Design review of the part built by this model. Coordinates are the model's own, in mm. A direction names the side the tool comes from. Coordinates: 2 decimals unless noted, no trailing zeros. Write each loop counter-clockwise with the first axis right and the second up, starting at its lowest first coordinate (ties: lowest second). Pieces come first, ordered by that corner, then holes.
```python
from build123d import *

# Parameters (mm, degrees)
SZKIC3_W                    = 1
SZKIC3_H                    = 17.528511895
WYTNIJ_WYCI_GNI_CIE1_DEPTH  = 35
WYTNIJ_WYCI_GNI_CIE4_DEPTH  = 12
SZKIC10_R                   = 6.25
DODANIE_WYCI_GNI_CIE5_DEPTH = 8
WYTNIJ_WYCI_GNI_CIE5_DEPTH  = 5
SZKIC12_R                   = 4
DODANIE_WYCI_GNI_CIE6_DEPTH = 23


with BuildPart() as part:
    # Szkic2 → Obrót1 (revolve)
    with BuildSketch(Plane(origin=(0, 0, 0), x_dir=(1, 0, 0), z_dir=(0, 1, 0))):
        Polygon((0, 0), (0, -40), (7, -53), (7, -63), (22, -63), (22, -40), (15, -40), (15, 0), align=None)
    revolve(axis=Axis((22, 0, 0), (0, 0, 1)))

    # Szkic3 → Wytnij-wyciągnięcie1 (cut)
    with BuildSketch(Plane(origin=(0, 0, 0), x_dir=(-1, 0, 0), z_dir=(0, 0, -1))):
        with Locations((-22, 13.789096025)):
            Rectangle(SZKIC3_W, SZKIC3_H)
    extrude(amount=-WYTNIJ_WYCI_GNI_CIE1_DEPTH, mode=Mode.SUBTRACT)

    # Szkic9 → Wytnij-wyciągnięcie4 (cut)
    with BuildSketch(Plane(origin=(0, 0, 0), x_dir=(0, 0, -1), z_dir=(1, 0, 0))):
        with BuildLine():
            Line((-2.956841624, 12.994317448), (-2.956841624, 31.011341841))
            Line((-2.956841624, 31.011341841), (-18.895064638, 31.011341841))
            Line((-18.895064638, 31.011341841), (-18.895064638, 12.002039571))
            ThreePointArc((-18.895064638, 12.002039571), (-10.459742092, 5.009776631), (-2.956841624, 12.994317448))
        make_face()
    extrude(amount=WYTNIJ_WYCI_GNI_CIE4_DEPTH, mode=Mode.SUBTRACT)

    # Szkic10 → Dodanie-wyciągnięcie5 (add)
    with BuildSketch(Plane.ZY.offset(-12)):
        with Locations(Location((10.956841624, 12.994317448, 0), (0, 0, 180))):
            Circle(SZKIC10_R)
    extrude(amount=DODANIE_WYCI_GNI_CIE5_DEPTH)

    # Szkic11 → Wytnij-wyciągnięcie5 (cut)
    with BuildSketch(Plane.ZY.offset(-4)):
        Polygon((14.360666712, 12.350908736), (13.215962457, 15.620412088), (9.812137369, 16.2638208), (7.553016536, 13.63772616), (8.697720791, 10.368222807), (12.101545879, 9.724814096), align=None)
    extrude(amount=-WYTNIJ_WYCI_GNI_CIE5_DEPTH, mode=Mode.SUBTRACT)

    # Szkic12 → Dodanie-wyciągnięcie6 (add)
    with BuildSketch(Plane.ZY.offset(-9)):
        with Locations((10.956841624, 12.994317448)):
            Circle(SZKIC12_R)
    extrude(amount=-DODANIE_WYCI_GNI_CIE6_DEPTH)


solid = part.part
```
(1) Insertion check: pin 1 Ø3.5 at (y, z) = (15.5, 9.5) entering from -X; pin 2 Ø6 at (y, z) = (-15, 45) entering from -X; pin 3 Ø11.5 at (y, z) = (15.5, 14.5) entering from -X. Each pin has a flat end and moves straight along its axis. Give the tip position at first contact, or say it passes through.
(2) Consider section C-C (z = 50.5). Give the boundary of the cut face in (x, y).
(3) Consider section B-B (z = 20.5). Give the boundary of the cut face in (x, y), plus the area to 3 significant figures.
(4) Consider section A-A (y = 0). Give the boundary of the cut face in (x, z).
(5) Wall thickness on line 1 (X direction, y = 0, z = 24.5); line 2 (Y direction, x = 22, z = 11); line 3 (Z direction, x = 9.5, y = 13): over which ranges is each line inside the solid? List them lowest first.
(6) For faces 4 (the cylindrical face through (36.985, -0.66, 58.07)), 5 (the flat face through (9, 16, 2.957)), 6 (the cylindrical face through (21.99, 14.2, 14.77)), 7 (the cylindrical face through (29, 0, 20)), 8 (the flat face through (6.465, 15.938, 11.538)), list the 3-axis set-ups (+Z, -Z, +X, -X, +Y, -Y) from which the entire face can be reached by the end or side of a thin tool; tool diameter is ignored.
(7) Mouldability with a two-part tool opening along Y and no side actions: class faces 1 (the flat face through (22, 0, 40)), 2 (the flat face through (4, 14, 14)), 3 (the cylindrical face through (38.215, -14.869, 20.28)) as +Y half, -Y half, draft (parallel to the pull), parting line (faces both ways), or undercut.
Results:
1. pin 1: stops at x = 4
1. pin 2: stops at x = 6.11
1. pin 3: stops at x = 3.4
2. outline: circle Ø32.69 at (22, 0)
3. outline: (21.5, 6.98) - (21.5, 21.99) arc R22 ccw (long way) to (22.5, 21.99) - (22.5, 6.98) arc R7 cw (long way) to start
3. area: 1,350 mm2
4. outline: (0, 0) - (15, 0) - (15, 40) - (29, 40) - (29, 0) - (44, 0) - (44, 40) - (37, 53) - (37, 63) - (7, 63) - (7, 53) - (0, 40) - close
5. line 1: x = 0 to 15, 29 to 44
5. line 2: y = -22 to -7, 8.99 to 16.99
5. line 3: z = 0 to 2.96, 4.71 to 17.21, 18.9 to 47.36
6. face 4: +Z
6. face 5: -X, +Y
6. face 6: none
6. face 7: -Z
6. face 8: -X
7. face 1: undercut
7. face 2: draft
7. face 3: parting line
